```python
from build123d import *

# Parameters (mm, degrees)
SKETCH_1_R      = 1.3
EXTRUDE_1_DEPTH = 3


with BuildPart() as part:
    # 草圖1 → 填料-伸長1 (new body)
    with BuildSketch(Plane.XY):
        with BuildLine():
            Line((216.492632944, 78.234092132), (216.493617135, 76.984092519))
            Line((216.493617135, 76.984092519), (213.99361791, 76.982124137))
            Line((213.99361791, 76.982124137), (213.992633719, 78.23212375))
            Line((213.992633719, 78.23212375), (210.000112684, 78.228980226))
            Line((210.000112684, 78.228980226), (209.999867004, 69.08))
            Line((209.999867004, 69.08), (223.48824264, 69.08))
            Line((223.48824264, 69.08), (237.517934203, 70.178792238))
            ThreePointArc((237.517934203, 70.178792238), (243.012429177, 75.673064936), (238.477244304, 81.982471062))
            Line((238.477244304, 81.982471062), (225.994777469, 84.991510945))
            Line((225.994777469, 84.991510945), (221.494778864, 84.987967857))
            Line((221.494778864, 84.987967857), (221.492416806, 87.987966928))
            Line((221.492416806, 87.987966928), (211.492419905, 87.980093399))
            Line((211.492419905, 87.980093399), (211.494781964, 84.980094329))
            Line((211.494781964, 84.980094329), (209.994782429, 84.9789133))
            Line((209.994782429, 84.9789133), (209.997745798, 81.228979292))
            Line((209.997745798, 81.228979292), (213.997733688, 81.232128695))
            Line((213.997733688, 81.232128695), (213.996749497, 82.482128308))
            Line((213.996749497, 82.482128308), (216.489286694, 82.484090815))
            Line((216.489286694, 82.484090815), (216.490270885, 81.234091202))
            Line((216.490270885, 81.234091202), (218.490270265, 81.235665908))
            Line((218.490270265, 81.235665908), (218.492632324, 78.235666838))
            Line((218.492632324, 78.235666838), (216.492632944, 78.234092132))
        make_face()
        with Locations((237.0017815, 76.100174585)):
            Circle(SKETCH_1_R, mode=Mode.SUBTRACT)
    extrude(amount=EXTRUDE_1_DEPTH)


solid = part.part
```
CAD build for the part. Positions are in the model's coordinates, mm. Round coordinates to 2 decimals unless told otherwise and drop trailing zeros. Order: outer loops, then holes, each group sorted by start corner. A loop starts at its lowest first (then second) coordinate and runs counter-clockwise, first axis right, second up.
Q1. Wall check: L1, parallel to Y at x = 218, z = 0.3; L2, parallel to X at y = 81.5, z = 2.4; L3, parallel to Y at x = 220, z = 2.2. Give the ranges that are in metal, low to high.
Q2. Slice it at A-A (z = 1.85). Write the cut outline in (x, y).
Q3. Two-plate mould, pull along X, no slides. Class faces 1 (the flat face through (232.323, 83.466, 1.479)), 2 (the flat face through (217, 69.08, 1)), 3 (the cylindrical face through (238.2, 75.6, 1.5)): pulls with the +X half, pulls with the -X half, needs draft (parallel to the pull), parting line crosses it, or undercut.
Q4. Slice it at B-B (x = 213.5). Write the cut outline in (y, z).
Q5. Slice it at C-C (y = 79). Write the cut outline in (x, z), and give its area (3 significant figures).
Q6. Slice it at D-D (x = 232.5). Write the cut outline in (y, z).
Q7. Drop flat-ended pins along their axis: pin 1 (1 mm diameter, centred on x = 226, y = 86, fed in from +Z); pin 2 (1 mm diameter, centred on y = 80, z = 2.5, fed in from +X). Give the stop position or say it passes through.
Results below:
1. L1: y = 69.08 to 78.24, 81.24 to 87.99
1. L2: x = 210 to 214, 216.49 to 239.77
1. L3: y = 69.08 to 87.99
2. outline: (209.99, 84.98) - (210, 81.23) - (214, 81.23) - (214, 82.48) - (216.49, 82.48) - (216.49, 81.23) - (218.49, 81.24) - (218.49, 78.24) - (216.49, 78.23) - (216.49, 76.98) - (213.99, 76.98) - (213.99, 78.23) - (210, 78.23) - (210, 69.08) - (223.49, 69.08) - (237.52, 70.18) arc R6 ccw to (238.48, 81.98) - (225.99, 84.99) - (221.49, 84.99) - (221.49, 87.99) - (211.49, 87.98) - (211.49, 84.98) - close; hole circle Ø2.6 at (237, 76.1)
3. face 1: pulls with the +X half
3. face 2: needs draft
3. face 3: undercut
4. outline: (69.08, 0) - (78.23, 0) - (78.23, 3) - (69.08, 3) - close; (81.23, 0) - (87.98, 0) - (87.98, 3) - (81.23, 3) - close
5. outline: (218.49, 0) - (242.32, 0) - (242.32, 3) - (218.49, 3) - close
5. area: 71.5 mm2
6. outline: (69.79, 0) - (83.42, 0) - (83.42, 3) - (69.79, 3) - close
7. pin 1: passes through
7. pin 2: stops at x = 242.02
